Source: three-view drawing plus pictorial views. Frame: mm from the lowest corner of the part. Give positions to 0.01 mm unless a question says otherwise; leave off trailing zeros. Order: outer loops, then holes, each group sorted by start corner. A loop starts at its lowest first (then second) coordinate and runs counter-clockwise, first axis right, second up. Notation, with made-up numbers: (-37.5, -20) - (-2.5, -20) arc R15 cw to (-2.5, 2) - close; hole circle Ø11 at (-21, 70). An arc over 180 degrees is marked (long way). Answer in a Markdown table with one row per item. Add a question column.
1. Section query C-C on y = 0.5. Count the separate pieces of the cut face and the enclosed holes in it, and give its area (3 significant figures).
2. Section query B-B on x = 14. Return loops of the section in (y, z).
3. Section query A-A on z = 20.5. Return loops of the section in (x, y).
4. Ray query, line 1 (Z direction, x = 5.75, y = 1.2); line 2 (X direction, y = 0.9, z = 20.5); line 3 (Z direction, x = 27, y = 0.2). Return the intervals inside material, ascending. Write a range as [from, to].
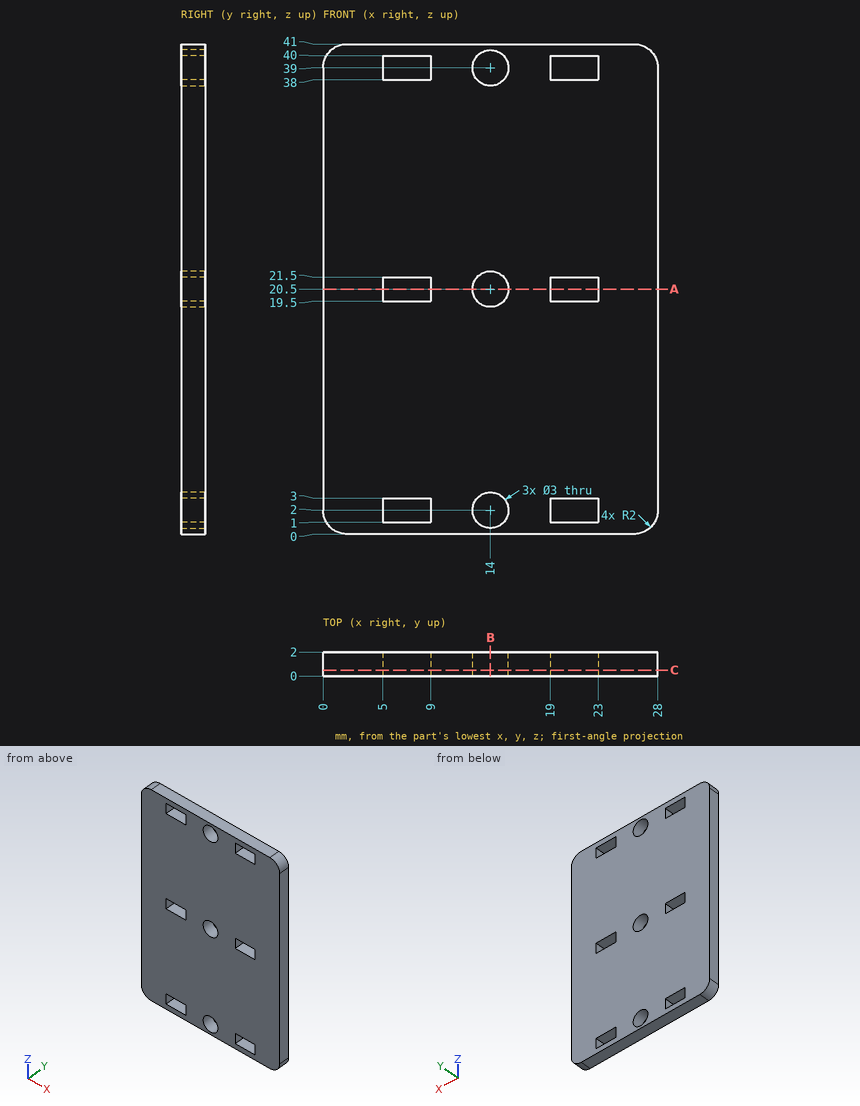
Answer:
| question | item | result |
|---|---|---|
| 1 | separate pieces | 1 |
| 1 | enclosed holes | 9 |
| 1 | area | 1,080 mm² |
| 2 | outline | (0, 0) - (2, 0) - (2, 0.5) - (0, 0.5) - close; (0, 3.5) - (2, 3.5) - (2, 19) - (0, 19) - close; (0, 22) - (2, 22) - (2, 37.5) - (0, 37.5) - close; (0, 40.5) - (2, 40.5) - (2, 41) - (0, 41) - close |
| 3 | outline | (0, 0) - (5, 0) - (5, 2) - (0, 2) - close; (9, 0) - (12.5, 0) - (12.5, 2) - (9, 2) - close; (15.5, 0) - (19, 0) - (19, 2) - (15.5, 2) - close; (23, 0) - (28, 0) - (28, 2) - (23, 2) - close |
| 4 | line 1 | z = [0, 1], [3, 19.5], [21.5, 38], [40, 41] |
| 4 | line 2 | x = [0, 5], [9, 12.5], [15.5, 19], [23, 28] |
| 4 | line 3 | z = [0.27, 40.73] |
